Source: CAD feature listing. Evaluate the final solid. Frame: model axes, mm. Face numbers are marked on the shaded views. Round coordinates to 2 decimals unless told otherwise and drop trailing zeros. Loops run counter-clockwise (first coordinate to the right, second up) from the corner with the lowest first, then second, coordinate; pieces in that order, holes last. Notation, with made-up numbers: (-23, 54) - (-8, 54) arc R22 cw to (-8, 92) - close; hole circle Ø2 at (18.5, 51). An arc over 180 degrees is marked (long way). One line per question, with ' | ' between items.
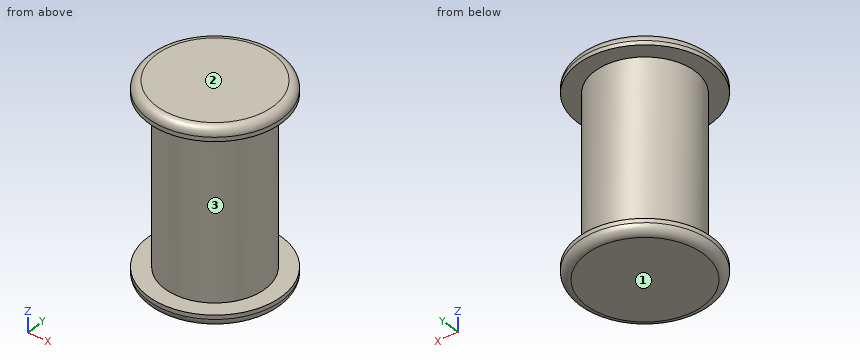
Autodesk Inventor part; units mm, degrees
ref_plane "YZ Plane" through (0, 0, 0) normal (1, 0, 0) x (0, 1, 0)
ref_plane "XZ Plane" through (0, 0, 0) normal (0, 1, 0) x (-1, 0, 0)
ref_plane "XY Plane" through (0, 0, 0) normal (0, 0, 1) x (1, 0, 0)
sketch "Sketch4" plane through (0, 0, 0) normal (1, 0, 0) x (0, 1, 0)
  line L0 (0, 0) -> (3, 0)
  line L1 (3, 0) -> (3, -5)
  line L2 (3, -5) -> (4, -5)
  line L3 (4, -5) -> (4, -5.75)
  line L4 (4, -5.75) -> (0, -5.75)
  line L5 (0, -5.75) -> (0, 0)
  dimension "d32" = 3
  dimension "d33" = 5
  dimension "d35" = 4
  dimension "d36" = 0.75
revolve "Revolution2" add sketch "Sketch4" angle 360 about axis through (0, 0, -5.75) along (0, 0, 1)
fillet "Fillet1" radius 0.5 1 edges at (0, -4, -5.75)
mirror "Mirror1" about plane through (0, 3, 0) normal (0, 0, 1) of "Revolution2", "Fillet1"
sketch "Boceto5" plane through (0, 0, 5.75) normal (0, 0, 1) x (1, 0, 0)
  circle A0 centre (0, 0) radius 3
properties part number "Sketch" material "Acero, alta resistencia, aleación baja"
1. Material intervals for probe 1 along Z at (x, y) = (-1.5, -3); probe 2 along X at (y, z) = (1.25, 4), sorted ascending.
Worked out:
probe 1: z = -5.75 to -5, 5 to 5.75 | probe 2: x = -2.73 to 2.73
2. Contact query for a flat-ended pin moving along its axis: P1, Ø2, axis at x = -1.5, z = -2.5, coming from the +Y side. Output: stop coordinate, or through.
Worked out:
P1: stops at y = 2.96
3. Section query C-C, the plane z = -4.5. Return loops of the section in (x, y).
Worked out:
outline: circle Ø6 at (0, 0)
4. Mould query, pull axis Z, two halves, no side actions, for the marked faces 1, 2 and 3. Classes: released by +Z, released by -Z, zero draft, split by the parting line, or undercut.
Worked out:
face 1: released by -Z | face 2: released by +Z | face 3: undercut
5. Section query A-A, the plane y = 0. Return loops of the section in (x, z).
Worked out:
outline: (-4, -5.25) arc R0.5 ccw to (-3.5, -5.75) - (3.5, -5.75) arc R0.5 ccw to (4, -5.25) - (4, -5) - (3, -5) - (3, 5) - (4, 5) - (4, 5.25) arc R0.5 ccw to (3.5, 5.75) - (-3.5, 5.75) arc R0.5 ccw to (-4, 5.25) - (-4, 5) - (-3, 5) - (-3, -5) - (-4, -5) - close
